Could you check a few things on this model? Use its own coordinates, in mm. Face numbers are marked on the shaded views. A direction names the side the tool comes from. Round coordinates to 2 decimals unless told otherwise and drop trailing zeros. Write each loop counter-clockwise with the first axis right and the second up, starting at its lowest first coordinate (ties: lowest second). Pieces come first, ordered by that corner, then holes. Notation, with made-up numbers: (36, 2) -> (75, 2) arc R14 cw to (75, 16) -> close; hole circle Ø4 at (-29, 27.25). An arc over 180 degrees is marked (long way). One line per question, with ' | ' between items. Start each with the question number.
1. Imagine slicing it at A-A, the plane x = 14. List the corners of the cut face in (y, z) for me, and give its area (3 significant figures).
2. If I drill on line 1 along X through (y, z) = (-0.6, -0.05); line 2 along Z through (x, y) = (4.5, -0.1); line 3 along X through (y, z) = (0, -1.4), over which ranges is the centre line in solid material (lowest first)? Write a range as [from, to].
3. For the marked faces 1 and 2, which set-ups out of +Z, -Z, +X, -X, +Y, -Y let a thin tool reach every point of the face, with its end or its side?
4. For pin 1 Ø0.6 at (x, z) = (-1, 0) entering from -Y; pin 2 Ø2 at (y, z) = (-1, 0) entering from +X, each with a flat end and sliding along its axis, tell me the tip position at first contact or that it passes through.
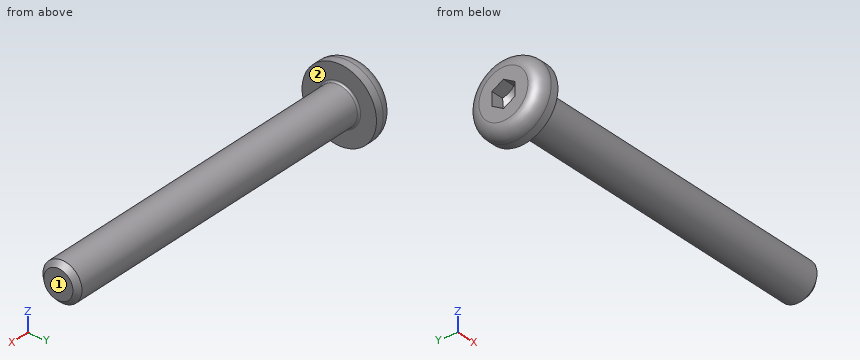
Autodesk Inventor part; units mm, degrees
ref_plane "Work Plane1" through (29, 0, 0) normal (0, -1, 0) x (1, 0, 0)
ref_plane "YZ Plane" through (0, 0, 0) normal (1, 0, 0) x (0, 1, 0)
ref_plane "XZ Plane" through (0, 0, 0) normal (0, 1, 0) x (-1, 0, 0)
sketch "Sketch1" plane through (0, 0, 0) normal (0, 0, 1) x (1, 0, 0)
  line L0 (-0.0254, 0) -> (19.05, 0)
  line L1 (19.05, 0) -> (19.05, 1.0922)
  line L2 (19.05, 1.0922) -> (1.016, 1.0922)
  line L3 (1.016, 1.0922) -> (0.1088, 1.0922)
  line L4 (0.1088, 1.0922) -> (0, 1.0922)
  line L5 (0, 1.0922) -> (0, 2.0828)
  line L6 (0, 2.0828) -> (-1.1684, 2.0828)
  line L7 (-1.1684, 2.0828) -> (-1.1684, 0.7479)
  line L8 (-1.1684, 0.7479) -> (-0.4572, 0.7479)
  line L9 (-0.4572, 0.7479) -> (-0.0254, 0)
  line L10 (-5.2121, 0) -> (23.0937, 0)
  line L11 (0, -0.4166) -> (0, 2.4994)
  line L12 (1.016, 1.0922) -> (0, 1.0922) construction
  dimension "d1" = 18.034
  dimension "d2" = 0.9072
  dimension "d3" = 1.1684
  dimension "d4" = 0.7112
  dimension "d5" = 60
  dimension "d6" = 2.1844
  dimension "d7" = 2.1844
  dimension "d8" = 1.4958
  dimension "d9" = 4.1656
  dimension "d26" = 19.05
revolve "Body" add sketch "Sketch1" angle 360 about axis through (-0.0254, 0, 0) along (1, 0, 0)
sketch "Sketch2" plane through (-1.1684, 0, 0) normal (-1, 0, 0) x (0, 0, 1)
  circle A0 centre (0, 0) radius 0.7479
  line L0 (0, -2.9159) -> (0, 2.9159)
  line L1 (-2.9159, 0) -> (2.9159, 0)
  line L2 (0.7479, 0) -> (0.3739, -0.6477)
  line L3 (0.3739, -0.6477) -> (-0.3739, -0.6477)
  line L4 (-0.3739, -0.6477) -> (-0.7479, 0)
  line L5 (-0.7479, 0) -> (-0.3739, 0.6477)
  line L6 (-0.3739, 0.6477) -> (0.3739, 0.6477)
  line L7 (0.3739, 0.6477) -> (0.7479, 0)
  point P0 (0, 0)
extrude "Slot" add sketch "Sketch2" against normal up to next contours L7 A0 | A0 L2 | L6 L0 A0 | A0 L0 L3 | L0 L6 A0 | A0 L3 L0 | L4 A0 | A0 L5
fillet "Fillet1" radius 0.7112 1 edges at (-1.1684, -2.0828, 0)
thread "Thread"
chamfer "Chamfer1" distance 0.2782 distance2 0.2781 1 edges at (19.05, -1.0922, 0) measured on face at (19.05, 0.3142, -0.0722)
ref_plane "Work Plane1" through (29, 0, 0) normal (0, -1, 0) x (1, 0, 0)
fillet "Fillet2" radius 0.1 1 edges at (0, -1.0922, 0)
equation "\"d1\" = GEL"
equation "\"d3\" = KOH"
equation "\"d4\" = INTI"
equation "\"d6\" = GD"
equation "\"d7\" = BDM"
equation "\"d8\" = 1.1547 * SW"
equation "\"d9\" = KOD"
equation "\"d26\" = NLG"
equation "\"d30\" = R"
equation "\"d17\" = RR"
equation "\"d13\" = GEL"
equation "\"d15\" = -0.5 * SPD + 0.5 * GD"
equation "\"d16\" = GUL"
equation "\"GD\" = NND"
equation "\"NLG\" = 19.05"
equation "\"GEL\" = 18.034"
equation "\"KOD\" = 4.1656"
equation "\"KOH\" = 1.1684"
equation "\"INTI\" = 0.7112"
equation "\"GAL\" = 0.90714"
equation "\"GUL\" = 0.27813"
equation "\"BDM\" = NND"
equation "\"SW\" = 1.2954"
equation "\"RR\" = 0.7112"
equation "\"SPD\" = GD1"
equation "\"R\" = 0.1"
equation "\"KR\" = 2.5146"
equation "\"GD1\" = 1.62793"
equation "\"THREADDIA\" = 2.1844"
equation "\"FAWI\" = 45deg"
equation "\"KOH1\" = 0.7112"
equation "\"NND\" = 2.1844"
equation "\"TOA\" = 30deg"
equation "\"E0\" = 1.155 * SW"
properties part number "Unbrako - 2 x 3/4" material "Steel, Mild"
Geometry results:
1) outline: circle Ø2.18 at (0, 0) | area: 3.75 mm2
2) line 1: x = [-0.37, 19.05] | line 2: z = [-1.09, 1.09] | line 3: x = [-1.17, 0]
3) face 1: +Z, -Z, +X, +Y, -Y | face 2: +X
4) pin 1: stops at y = -2.04 | pin 2: stops at x = 19.05
